Geometry check sheet. Reference: the model listing, model coordinates, mm. A direction names the side the tool comes from. Coordinates: 2 decimals unless noted, no trailing zeros. Write each loop counter-clockwise with the first axis right and the second up, starting at its lowest first coordinate (ties: lowest second). Pieces come first, ordered by that corner, then holes. Notation, with made-up numbers: (73.25, 87) -> (85.25, 87) arc R20 cw to (85.25, 93) -> close; hole circle Ø3 at (2, 41). An arc over 180 degrees is marked (long way). Answer in a Markdown table with one row per item. Add a question column.
Q1. Section check D-D, the plane z = 12.25. Record the boundary of the cut face in (x, y), and give its area (3 significant figures).
Q2. Thickness scan on line 1 (Y direction, x = 0.5, z = 23); line 2 (Z direction, x = -7.5, y = 8); line 3 (Y direction, x = 12, z = 24.5). Record the ranges inside material, lowest first.
Q3. Tool access check on faces 1 (the face through (0, 0, 0)), 2 (the face through (-2.17, 9.76, 3.54)). Record the directions out of +Z, -Z, +X, -X, +Y, -Y that give a thin tool (end or side, any length) a straight path to the whole face; none if there is none.
Q4. Section check A-A, the plane x = 0. Record the boundary of the cut face in (y, z), and give its area (3 significant figures).
Q5. Section check C-C, the plane z = 5.25. Record the boundary of the cut face in (x, y), and give its area (3 significant figures).
Q6. Gauge pin test, flat ends, axial feed: P1, Ø1, axis at x = -5, z = 17.5, coming from the -Y side; P2, Ø1.5, axis at x = -10, z = 18.5, coming from the +Y side; P3, Ø3, axis at y = 8, z = 9, coming from the -X side; P4, Ø8, axis at x = 6, y = 2.5, coming from the -Z side. Record the tip position at first contact, or that the pin passes through.
```python
from build123d import *


with BuildPart() as f1:
    # F0 (on Front) → F1 (revolve)
    with BuildSketch(Plane.XZ):
        with BuildLine():
            Line((9, 0), (10, 1))
            Line((10, 1), (10, 6))
            Line((10, 6), (11, 6))
            ThreePointArc((11, 6), (13.828427, 7.171573), (15, 10))
            Line((15, 10), (15, 24.5))
            ThreePointArc((15, 24.5), (13.828427, 27.328427), (11, 28.5))
            Line((11, 28.5), (0, 28.5))
            Line((0, 28.5), (0, 0))
            Line((0, 0), (9, 0))
        make_face()
    revolve(axis=Axis((0, 0, 14.25), (0, 0, -1)))


solid = f1.part
```
Calculated:
| question | item | result |
|---|---|---|
| 1 | outline | circle Ø30 at (0, 0) |
| 1 | area | 707 mm² |
| 2 | line 1 | y = -14.99 to 14.99 |
| 2 | line 2 | z = 6 to 28.5 |
| 2 | line 3 | y = -9 to 9 |
| 3 | face 1 | -Z, +X, -X, +Y, -Y |
| 3 | face 2 | -Z |
| 4 | outline | (-15, 10) arc R4 ccw to (-11, 6) -> (-10, 6) -> (-10, 1) -> (-9, 0) -> (9, 0) -> (10, 1) -> (10, 6) -> (11, 6) arc R4 ccw to (15, 10) -> (15, 24.5) arc R4 ccw to (11, 28.5) -> (-11, 28.5) arc R4 ccw to (-15, 24.5) -> close |
| 4 | area | 780 mm² |
| 5 | outline | circle Ø20 at (0, 0) |
| 5 | area | 314 mm² |
| 6 | P1 | stops at y = -14.31 |
| 6 | P2 | stops at y = 11.81 |
| 6 | P3 | stops at x = -13.44 |
| 6 | P4 | stops at z = 0 |
